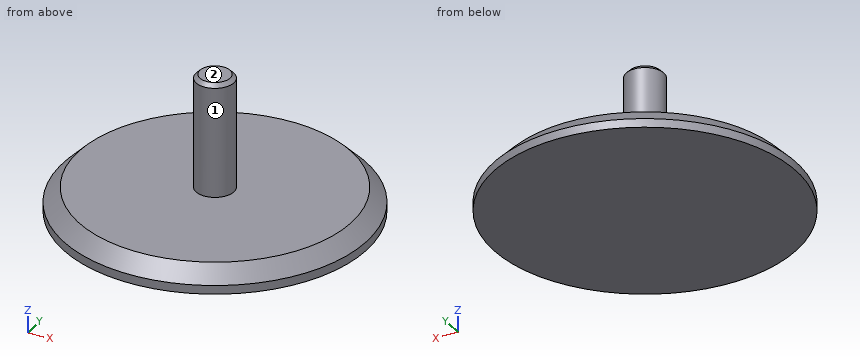
from build123d import *

# Parameters (mm, degrees)
F0_R     = 1.27
F1_DEPTH = 7.62
F2_R     = 10.16
F3_DEPTH = 1.6002
F4_SIZE  = 1.016
F5_SIZE  = 0.254


with BuildPart() as f1:
    # F0 (on Top) → F1 (new body)
    with BuildSketch(Plane.XY):
        Circle(F0_R)
    extrude(amount=-F1_DEPTH)

    # F2 (on face) → F3 (join)
    with BuildSketch(Plane(origin=(0, 0, -7.62), x_dir=(1, 0, 0), z_dir=(0, 0, -1))):
        Circle(F2_R)
    extrude(amount=F3_DEPTH)

    # F4
    f4_edges = [f1.edges().sort_by_distance(p)[0] for p in [
        (-10.16, 0, -7.62),
    ]]
    chamfer(f4_edges, length=F4_SIZE)

    # F5
    f5_edges = [f1.edges().sort_by_distance(p)[0] for p in [
        (-1.27, 0, 0),
    ]]
    chamfer(f5_edges, length=F5_SIZE)


solid = f1.part
Verification items for the finished model (mm, model axes). Face numbers are marked on the shaded views. A direction names the side the tool comes from. Give positions to 0.01 mm unless a question says otherwise; leave off trailing zeros. Write each loop counter-clockwise with the first axis right and the second up, starting at its lowest first coordinate (ties: lowest second). Pieces come first, ordered by that corner, then holes. Notation, with made-up numbers: (63.25, -8.5) - (113.25, -8.5) arc R22 ccw to (113.25, 7.5) - close; hole circle Ø9 at (40.25, -38.75). An arc over 180 degrees is marked (long way). Answer as CSV lines item,"result". Start each with the question number.
1. Sectioned sample at D-D (z = -8.25). Record the boundary of the cut face in (x, y), then the cut area to 3 significant figures.
2. Sectioned sample at C-C (z = -6). Record the boundary of the cut face in (x, y), then the cut area to 3 significant figures.
3. Depth check by flat-ended pin: pin 1 (1 mm diameter, centred on x = -0.5, y = 2.5, fed in from +Z); pin 2 (3 mm diameter, centred on y = 2.5, z = -2, fed in from -X); pin 3 (1.5 mm diameter, centred on x = 1.5, z = -8, fed in from -Y). Enter the tip coordinate at first touch or a pass-through.
4. Set-up check for the marked faces 1 and 2: record each of +Z, -Z, +X, -X, +Y, -Y from which the full face is reachable in a straight line by a thin tool's end or side.
5. Thickness scan on line 1 (Z direction, x = 2, y = 0.5); line 2 (X direction, y = -0.5, z = -5); line 3 (Y direction, x = 0.25, z = -5.25). Record the ranges inside material, lowest first.
6. Sectioned sample at A-A (x = 0). Record the boundary of the cut face in (y, z).
Derived:
1,outline,"circle Ø19.55 at (0, 0)"
1,area,"300 mm²"
2,outline,"circle Ø2.54 at (0, 0)"
2,area,"5.07 mm²"
3,pin 1,"z = -7.62"
3,pin 2,"x = -0.78"
3,pin 3,"y = -10.1"
4,face 1,"+Z"
4,face 2,"+Z, +X, -X, +Y, -Y"
5,line 1,"-9.22 to -7.62"
5,line 2,"-1.17 to 1.17"
5,line 3,"-1.25 to 1.25"
6,outline,"(-10.16, -9.22) - (10.16, -9.22) - (10.16, -8.64) - (9.14, -7.62) - (1.27, -7.62) - (1.27, -0.25) - (1.02, 0) - (-1.02, 0) - (-1.27, -0.25) - (-1.27, -7.62) - (-9.14, -7.62) - (-10.16, -8.64) - close"
